```python
from build123d import *

# Parameters (mm, degrees)
F2_W     = 37.1675528586
F2_H     = 166.4876639843
F3_DEPTH = 82.2
F4_W     = 40.7858882099
F4_H     = 148.783929646
F5_DEPTH = 98.6


with BuildPart() as f1:
    # F0 (on Top) → F1 (revolve)
    with BuildSketch(Plane.XY):
        Polygon((-19.6189273595, 46.4221443981), (-59.5299630911, 46.4221443981), (-59.5299630911, 3.069964936), (147.5333869457, 0), (147.9226052761, 20.7655709237), (125.3759115934, 20.7655709237), (125.3759115934, 40.7577455044), (97.2828418016, 40.7577455044), (97.2828418016, 47.2125634551), (68.3147385716, 47.2125634551), (68.3147385716, 40.7577455044), (48.1183305383, 40.7577455044), (48.1183305383, 34.2763438821), (20.6776820123, 34.2763438821), (20.6776820123, 27.4582132697), (-19.6189273595, 27.4582132697), align=None)
    revolve(axis=Axis((44.0017119273, 1.534982468, 0), (0.9998901098, -0.0148245818, 0)))

    # F2 (on Front) → F3 (cut)
    with BuildSketch(Plane.XZ):
        with Locations((-18.5837764293, 5.1509216428)):
            Rectangle(F2_W, F2_H)
    extrude(amount=-F3_DEPTH, mode=Mode.SUBTRACT)

    # F4 (on Front) → F5 (cut)
    with BuildSketch(Plane.XZ):
        with Locations((47.2418097779, -5.5372081697)):
            Rectangle(F4_W, F4_H)
    extrude(amount=F5_DEPTH, mode=Mode.SUBTRACT)


solid = f1.part
```
Model file for the job. Use its own axes, mm. A direction names the side the tool comes from. Coordinates: 2 decimals unless noted, no trailing zeros. Answer as a JSON object with one key per item and string values. Group by question number.
1) Cut at A-A, the plane y = -28.5. Count the separate pieces of the cut face and the enclosed holes in it, then the cut area to 3 significant figures.
2) Which spindle directions (+Z, -Z, +X, -X, +Y, -Y) get a long thin tool onto all of the face, cutting with end or side? Do faces 3 (the face through (-20.395, -23.671, 0.555)), 4 (the face through (-23, 0, 1)), 5 (the face through (136.12, -4.3, -20.11)), 6 (the face through (26.849, -12, 0)), 7 (the face through (-45.58, -40.673, 1.916)). Say none if no direction does.
3) Pull direction X, two halves, no side cores. Call faces 1 (the face through (147.534, -0.282, -1.268)), 2 (the face through (20.21, -3.73, -25.29)): +X half, -X half, draft (parallel to the pull), parting line (faces both ways), or undercut.
4) Flat gauge pins, fed straight in: pin 1 (4 mm diameter, centred on y = -12, z = -23, fed in from +X); pin 2 (5 mm diameter, centred on x = -36, z = 24, fed in from +Y); pin 3 (8 mm diameter, centred on x = 67, y = -9, fed in from -Z). Where does each tip first touch, or does it go through?
5) Drill centre lines: L1, parallel to X at y = 31.5, z = -10.5; L2, parallel to X at y = -9, z = -30; L3, parallel to X at y = 23.5, z = 14.5. Where is each one in solid material? Low to high.
Check values:
{
 "1": {"separate pieces": "3", "enclosed holes": "0", "area": "6,200 mm²"},
 "2": {"face 3": "-Y", "face 4": "+Z, -Z, +Y", "face 5": "none", "face 6": "+Z, -Z, -Y", "face 7": "-X"},
 "3": {"face 1": "+X half", "face 2": "undercut"},
 "4": {"pin 1": "stops at x = 124.86", "pin 2": "stops at y = 40.6", "pin 3": "stops at z = -45.61"},
 "5": {"L1": "x = -59.56 to -37.17, 20.65 to 125.35", "L2": "x = -60.19 to -20.27, 20.04 to 26.85, 67.63 to 124.77", "L3": "x = -59.6 to -37.17, 20.61 to 125.31"}
}
